```python
from build123d import *

# Parameters (mm, degrees)
F0_W     = 40
F0_H     = 50
F0_R     = 2.5
F0_W_2   = 10
F0_W_3   = 5
F0_H_2   = 45
F1_DEPTH = 5


with BuildPart() as f1:
    # F0 (on Top) → F1 (new body)
    with BuildSketch(Plane.XY):
        Rectangle(F0_W, F0_H)
        with Locations((14, -7.681146)):
            Circle(F0_R, mode=Mode.SUBTRACT)
        with Locations((-15, 0)):
            Circle(F0_R, mode=Mode.SUBTRACT)
        with Locations((14, 7.681146)):
            Circle(F0_R, mode=Mode.SUBTRACT)
        with Locations((15, 0)):
            Circle(F0_R, mode=Mode.SUBTRACT)
        with Locations((-25, 0)):
            Rectangle(F0_W_2, F0_H)
        with Locations((-25, 0)):
            Rectangle(F0_W_3, F0_H_2, mode=Mode.SUBTRACT)
        with Locations((25, 0)):
            Rectangle(F0_W_2, F0_H)
        with Locations((25, 0)):
            Rectangle(F0_W_3, F0_H_2, mode=Mode.SUBTRACT)
    extrude(amount=F1_DEPTH)


solid = f1.part
```
Part model, mm, in its own coordinate system. A direction names the side the tool comes from. Round coordinates to 2 decimals unless told otherwise and drop trailing zeros. Write each loop counter-clockwise with the first axis right and the second up, starting at its lowest first coordinate (ties: lowest second). Pieces come first, ordered by that corner, then holes.
Item 1: Cut at C-C, the plane x = 15. Give the cut face in (y, z), plus the area to 3 significant figures.
Results:
outline: (-25, 0) - (-9.97, 0) - (-9.97, 5) - (-25, 5) - close; (-5.39, 0) - (-2.5, 0) - (-2.5, 5) - (-5.39, 5) - close; (2.5, 0) - (5.39, 0) - (5.39, 5) - (2.5, 5) - close; (9.97, 0) - (25, 0) - (25, 5) - (9.97, 5) - close
area: 179 mm2
Item 2: Which spindle directions (+Z, -Z, +X, -X, +Y, -Y) get a long thin tool onto all of the face, cutting with end or side? Do faces 5 (the flat face through (0, 0, 5)), 6 (the flat face through (22.5, 0, 2)). Say none if no direction does.
Results:
face 5: +Z, +X, -X, +Y, -Y
face 6: +Z, -Z
Item 3: Probe L1, parallel to X at y = -4, z = 0.9; L2, parallel to Y at x = 15, z = 2.35; L3, parallel to Y at x = 27, z = 3.55. List the from-to ranges inside material, lowest first.
Results:
L1: x = -30 to -27.5, -22.5 to 22.5, 27.5 to 30
L2: y = -25 to -9.97, -5.39 to -2.5, 2.5 to 5.39, 9.97 to 25
L3: y = -25 to -22.5, 22.5 to 25
Item 4: Cut at D-D, the plane y = 9.5. Give the cut face in (x, z).
Results:
outline: (-30, 0) - (-27.5, 0) - (-27.5, 5) - (-30, 5) - close; (-22.5, 0) - (12.28, 0) - (12.28, 5) - (-22.5, 5) - close; (15.72, 0) - (22.5, 0) - (22.5, 5) - (15.72, 5) - close; (27.5, 0) - (30, 0) - (30, 5) - (27.5, 5) - close
Item 5: Two-plate mould, pull along Y, no slides. Class faces 1 (the flat face through (0, 0, 0)), 2 (the flat face through (0, 25, 2)), 3 (the flat face through (0, -25, 2)), 4 (the cylindrical face through (11.502, 7.791, 2.465)): +Y half, -Y half, draft (parallel to the pull), parting line (faces both ways), or undercut.
Results:
face 1: draft
face 2: +Y half
face 3: -Y half
face 4: undercut
Item 6: Cut at A-A, the plane y = -4. Give the cut face in (x, z).
Results:
outline: (-30, 0) - (-27.5, 0) - (-27.5, 5) - (-30, 5) - close; (-22.5, 0) - (22.5, 0) - (22.5, 5) - (-22.5, 5) - close; (27.5, 0) - (30, 0) - (30, 5) - (27.5, 5) - close
Item 7: Cut at B-B, the plane x = -26. Give the cut face in (y, z), plus the area to 3 significant figures.
Results:
outline: (-25, 0) - (-22.5, 0) - (-22.5, 5) - (-25, 5) - close; (22.5, 0) - (25, 0) - (25, 5) - (22.5, 5) - close
area: 25.0 mm2
